Can you work these out from the drawing? Everything is in mm from the part's minimum corner. Round coordinates to 2 decimals unless told otherwise and drop trailing zeros. Write each loop counter-clockwise with the first axis right and the second up, starting at its lowest first coordinate (ties: lowest second). Pieces come first, ordered by that corner, then holes. Notation, with made-up numbers: (-17, 4) - (4, 4) arc R18 ccw to (4, 9) - close; hole circle Ø3 at (-14, 3). An arc over 180 degrees is marked (long way). One line per item, written item: value. Start each with the question number.
Item 1: Imagine slicing it at C-C, the plane x = 42.5. Please give me the cut outline in (y, z) (1 decimal), then the cut area to 3 significant figures.
Item 2: If I drill on line 1 (Y direction, x = 71, z = 42.5); line 2 (Y direction, x = 70.5, z = 44); line 3 (X direction, y = 41, z = 29) (1 decimal), over which ranges is the centre line in solid material (lowest first)?
Item 3: Imagine slicing it at A-A, the plane x = 79. Please give me the cut outline in (y, z) (1 decimal).
Item 4: Imagine slicing it at D-D, the plane y = 21.5. Please give me the cut outline in (x, z).
Item 5: Thinking about a two-plate mould opening in X: for the marked faces 1, 2, 3 and 4, which applies, released by +X, released by -X, zero draft, split by the parting line, or undercut?
Item 6: Imagine slicing it at B-B, the plane z = 41. Please give me the cut outline in (x, y) (1 decimal).
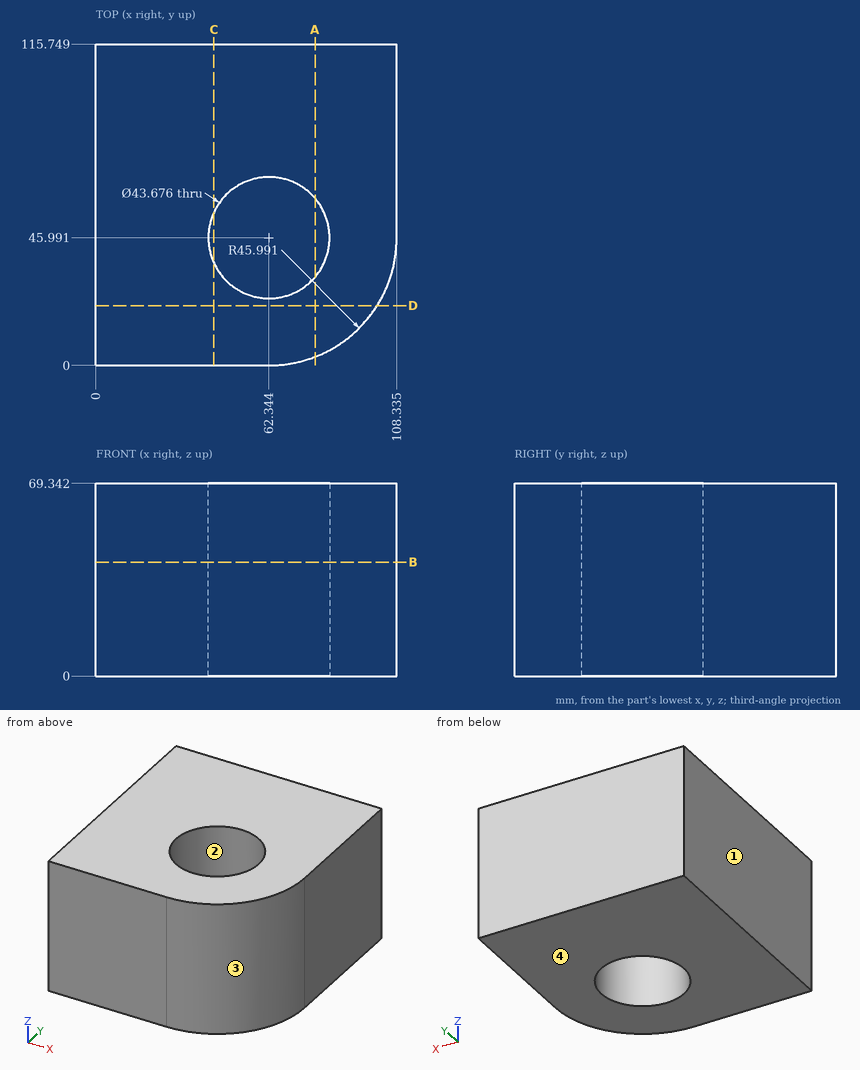
Values follow:
1. outline: (0, 0) - (36.9, 0) - (36.9, 69.3) - (0, 69.3) - close; (55.1, 0) - (115.7, 0) - (115.7, 69.3) - (55.1, 69.3) - close
1. area: 6,760 mm^2
2. line 1: y = 0.82 to 25.94, 66.04 to 115.75
2. line 2: y = 0.73 to 25.73, 66.25 to 115.75
2. line 3: x = 0 to 41.1, 83.6 to 108.1
3. outline: (3.1, 0) - (31.9, 0) - (31.9, 69.3) - (3.1, 69.3) - close; (60.1, 0) - (115.7, 0) - (115.7, 69.3) - (60.1, 69.3) - close
4. outline: (0, 0) - (101.27, 0) - (101.27, 69.34) - (0, 69.34) - close
5. face 1: released by -X
5. face 2: undercut
5. face 3: released by +X
5. face 4: zero draft
6. outline: (0, 0) - (62.3, 0) arc R46 ccw to (108.3, 46) - (108.3, 115.7) - (0, 115.7) - close; hole circle Ø43.7 at (62.3, 46)
